Check sheet for the modelled part. Datum: model origin and axes. Units: mm. A direction names the side the tool comes from. Round coordinates to 2 decimals unless told otherwise and drop trailing zeros. Write each loop counter-clockwise with the first axis right and the second up, starting at its lowest first coordinate (ties: lowest second). Pieces come first, ordered by that corner, then holes.
Item 1: Material ranges on line 1 along Y through (x, z) = (116.75, 16.25); line 2 along Z through (x, y) = (117.5, 12.25), recorded low to high.
Item 2: Section check A-A, the plane y = 12.8. Record the cut outline in (x, z).
Item 3: Depth check by flat-ended pin: pin 1 (1.6 mm diameter, centred on x = 116.5, y = 13, fed in from +Z); pin 2 (1.6 mm diameter, centred on x = 116.75, y = 12.8, fed in from +Z). Enter the tip coordinate at first touch or a pass-through.
Item 4: Release check for a two-part mould opening along X. For faces 1 (the cylindrical face through (117.675, 13.091, 15.965)), 2 (the flat face through (118.5, 13, 12)), 3 (the flat face through (116, 13, 5)) record: pulls with the +X half, pulls with the -X half, needs draft (parallel to the pull), parting line crosses it, or undercut.
Item 5: Set-up check for faces 4 (the flat face through (117, 13, 13.5)), 5 (the flat face through (115, 13, 18.5)): record each of +Z, -Z, +X, -X, +Y, -Y from which the full face is reachable in a straight line by a thin tool's end or side.
Item 6: Section check B-B, the plane x = 116.75. Record the cut outline in (y, z), plus the area to 3 significant figures.
Item 7: Section check C-C, the plane z = 14.5. Record the cut outline in (x, y).
from build123d import *

# Parameters (mm, degrees)
CYLINDER002002001001001001001001007_R     = 0.97
CYLINDER002002001001001001001001007_DEPTH = 5
BOX006001_W                               = 4.5
BOX006001_H                               = 10
BOX006001_DEPTH                           = 13.5


with BuildPart() as cylinder002002001001001001001001007:
    # Cylinder002002001001001001001001007 → Cylinder002002001001001001001001007 (new body)
    with BuildSketch(Plane(origin=(116.75, 12.8, 13.5), x_dir=(1, 0, 0), z_dir=(0, 0, 1))):
        Circle(CYLINDER002002001001001001001001007_R)
    extrude(amount=CYLINDER002002001001001001001001007_DEPTH)


with BuildPart() as cut013003022:
    # Box006001 → Box006001 (new body)
    with BuildSketch(Plane(origin=(114, 7.8, 5), x_dir=(1, 0, 0), z_dir=(0, 0, 1))):
        with Locations((2.25, 5)):
            Rectangle(BOX006001_W, BOX006001_H)
    extrude(amount=BOX006001_DEPTH)

    # Cut013003022: cut Cylinder002002001001001001001001007
    add(cylinder002002001001001001001001007.part, mode=Mode.SUBTRACT)


solid = cut013003022.part
Values found:
1. line 1: y = 7.8 to 11.83, 13.77 to 17.8
1. line 2: z = 5 to 13.5
2. outline: (114, 5) - (118.5, 5) - (118.5, 18.5) - (117.72, 18.5) - (117.72, 13.5) - (115.78, 13.5) - (115.78, 18.5) - (114, 18.5) - close
3. pin 1: stops at z = 18.5
3. pin 2: stops at z = 13.5
4. face 1: undercut
4. face 2: pulls with the +X half
4. face 3: needs draft
5. face 4: +Z
5. face 5: +Z, +X, -X, +Y, -Y
6. outline: (7.8, 5) - (17.8, 5) - (17.8, 18.5) - (13.77, 18.5) - (13.77, 13.5) - (11.83, 13.5) - (11.83, 18.5) - (7.8, 18.5) - close
6. area: 125 mm2
7. outline: (114, 7.8) - (118.5, 7.8) - (118.5, 17.8) - (114, 17.8) - close; hole circle Ø1.94 at (116.75, 12.8)
